Work out the finished part from the listing and answer in its coordinate system (mm). Round coordinates to 2 decimals unless told otherwise and drop trailing zeros. Loops run counter-clockwise (first coordinate to the right, second up) from the corner with the lowest first, then second, coordinate; pieces in that order, holes last. Notation, with made-up numbers: (-32, -24.5) - (-14, -24.5) arc R26 cw to (-14, -8.5) - close; hole circle Ø7 at (13.5, 40). An arc over 180 degrees is marked (long way). Return JSON: item names as keys, results as strings.
from build123d import *

# Parameters (mm, degrees)
BOSS_EXTRU_1_DEPTH = 10
CONG_2_R           = 10


with BuildPart() as part:
    # Esquisse1 → Boss.-Extru.1 (new body)
    with BuildSketch(Plane(origin=(0, 0, 0), x_dir=(1, 0, 0), z_dir=(0, 1, 0))):
        Polygon((0, 0), (70, 0), (70, -100), (40, -100), (30, -100), (0, -100), align=None)
    extrude(amount=BOSS_EXTRU_1_DEPTH)

    # Congé2
    cong_2_edges = [part.edges().sort_by_distance(p)[0] for p in [
        (0, 5, 0),
        (70, 5, 0),
        (70, 5, 100),
        (0, 5, 100),
    ]]
    fillet(cong_2_edges, radius=CONG_2_R)


solid = part.part
1) Section A-A (z = 93.5) is taken. Give the vertices of the cut face in (x, y), and give its area (3 significant figures).
Verdict:
{"outline": "(0.63, 0) - (69.37, 0) - (69.37, 10) - (0.63, 10) - close", "area": "687 mm2"}
2) Find the intervals of material crossed by L1, parallel to Z at x = 60.5, y = 8.25; L2, parallel to Z at x = 5.5, y = 9.25; L3, parallel to X at y = 9.5, z = 94, in increasing order.
Verdict:
{"L1": "z = 0.01 to 99.99", "L2": "z = 1.07 to 98.93", "L3": "x = 0.83 to 69.17"}
3) Determine the mould class of faces 1 (the cylindrical face through (3.01, 5.07, 97.15)), 2 (the flat face through (70, 5, 49)), 3 (the cylindrical face through (66.99, 5.07, 2.85)) for opening direction Z: pulls with the +Z half, pulls with the -Z half, needs draft (parallel to the pull), parting line crosses it, or undercut.
Verdict:
{"face 1": "pulls with the +Z half", "face 2": "needs draft", "face 3": "pulls with the -Z half"}
4) Section B-B (x = 5) is taken. Give the vertices of the cut face in (y, z).
Verdict:
{"outline": "(0, 1.34) - (10, 1.34) - (10, 98.66) - (0, 98.66) - close"}
